Autodesk Inventor part; units mm, degrees
ref_plane "YZ Plane" through (0, 0, 0) normal (1, 0, 0) x (0, 1, 0)
ref_plane "XZ Plane" through (0, 0, 0) normal (0, 1, 0) x (-1, 0, 0)
ref_plane "XY Plane" through (0, 0, 0) normal (0, 0, 1) x (1, 0, 0)
sketch "スケッチ1" plane through (0, 0, 0) normal (0, 0, 1) x (1, 0, 0)
  line L0 (-5.9, -14.9) -> (5.9, -14.9) construction
  line L1 (5.9, -14.9) -> (5.9, 14.9) construction
  line L2 (5.9, 14.9) -> (-5.9, 14.9) construction
  line L3 (-5.9, 14.9) -> (-5.9, -14.9) construction
  line L4 (-5.9, -14.9) -> (5.9, 14.9) construction
  line L5 (5.9, -14.9) -> (-5.9, 14.9) construction
  circle A0 centre (-5.9, 14.9) radius 1.1
  circle A1 centre (-5.9, 14.9) radius 2
  circle A2 centre (5.9, 14.9) radius 2
  circle A3 centre (5.9, 14.9) radius 1.1
  circle A4 centre (-5.9, -14.9) radius 2
  circle A5 centre (-5.9, -14.9) radius 1.1
  circle A6 centre (5.9, -14.9) radius 2
  circle A7 centre (5.9, -14.9) radius 1.1
  circle A8 centre (0, 8.9998) radius 6.5
  circle A9 centre (-5.9, 14.9) radius 8.344 construction
  line L6 (-6.5, 8.9998) -> (6.5, 8.9998)
  line L7 (6.5, 8.9998) -> (6.5, -11.9)
  line L8 (6.5, -11.9) -> (-6.5, -11.9)
  line L9 (-6.5, -11.9) -> (-6.5, 8.9998)
  line L10 (-7.9, -16.9) -> (7.9, -16.9)
  line L11 (7.9, -16.9) -> (7.9, 16.9)
  line L12 (7.9, 16.9) -> (-7.9, 16.9)
  line L13 (-7.9, 16.9) -> (-7.9, -16.9)
  line L14 (-7.9, -16.9) -> (7.9, 16.9) construction
  line L15 (7.9, -16.9) -> (-7.9, 16.9) construction
  line L16 (-15.25, -0.0002) -> (15.25, -0.0002)
  line L17 (15.25, -0.0002) -> (15.25, 17.9998)
  line L18 (15.25, 17.9998) -> (-15.25, 17.9998)
  line L19 (-15.25, 17.9998) -> (-15.25, -0.0002)
  line L20 (-15.25, -0.0002) -> (15.25, 17.9998) construction
  line L21 (15.25, -0.0002) -> (-15.25, 17.9998) construction
  point P0 (0, 0)
  point P1 (0, 14.9)
  point P2 (7.9, -0.0002)
  point P3 (-7.9, -0.0002)
  point P4 (-7.9, -14.9)
  point P5 (-5.9, -16.9)
  point P6 (5.9, -16.9)
  point P7 (7.9, -14.9)
  point P8 (6.5, 8.9998)
  dimension "d12" = 13
  dimension "d13" = 16.688
  dimension "d0" = 11.8
  dimension "d1" = 29.8
  dimension "d2" = 2.2
  dimension "d3" = 4
  dimension "d6" = 11.8
  dimension "d9" = 29.8
  dimension "d14" = 3
  dimension "d15" = 30.5
  dimension "d16" = 18
extrude "押し出し1" add sketch "スケッチ1" along normal blind 3 contours A1 A8 | A1 L12 A2 A8 | L12 L13 L16 L19 L18 L17 L11 | A1 L13 L12 | A1 A8 L9 L16 L13 | L12 L11 A2 | A2 A8 | L16 L9 L8 L7 L11 A6 L10 A4 L13 | L11 L16 L7 A8 A2 | A4 | A6 picked at (-7.5833, 15.0483) picked at (7.5833, 15.0483)
fillet "フィレット1" radius 2 4 edges at (-7.9, -0.0002, 1.5) (7.9, -0.0002, 1.5) (-6.5, -11.9, 1.5) (6.5, -11.9, 1.5)
sketch "スケッチ2" plane through (-15.25, -0.0002, 0) normal (-1, 0, 0) x (0, 0, 1)
  line L0 (0, 18) -> (3, 18) construction
  line L1 (1.5, 18) -> (1.5, 0) construction
  line L2 (0, 0) -> (3, 0) construction
  line L3 (0, 9) -> (3, 9) construction
  line L4 (1.5, 9) -> (3, 9) construction
  point P0 (0, 0.0002)
  point P1 (1.5, 16.5)
  point P2 (1.5, 1.5)
  dimension "d20" = 15
hole "穴1" at (-15.25, 16.4998, 1.5) at (-15.25, 1.4998, 1.5) direction (1, 0, 0) diameter 1.567 depth 4.5 tip angle 118
sketch "スケッチ3" plane through (15.25, -0.0002, 0) normal (1, 0, 0) x (0, 0, -1)
  line L0 (0, 0) -> (0, 18)
  circle A0 centre (-1.5, 1.5) radius 0.7835
  circle A1 centre (-1.5, 16.5) radius 0.7835
  line L1 (0, 18) -> (0, 0)
  line L2 (0, 0) -> (-3, 0)
  line L3 (-3, 18) -> (-3, 0)
  line L4 (0, 18) -> (-3, 18)
  point P0 (0, 0.0002)
hole "穴2" at (15.25, 1.4998, 1.5) at (15.25, 16.4998, 1.5) direction (-1, 0, 0) diameter 1.567 depth 4.5 tip angle 118
sketch "スケッチ4" plane through (0, 0, 3) normal (0, 0, 1) x (1, 0, 0)
  line L0 (-15.25, 0.7163) -> (-15.25, 2.2833)
  line L1 (-15.25, 15.7163) -> (-15.25, 17.2833)
  circle A0 centre (-16.15, 1.4998) radius 1.1
  line L2 (-15.25, 17.9998) -> (-15.25, -0.0002) construction
  line L3 (-15.25, 8.9998) -> (15.25, 8.9998) construction
  line L4 (15.25, -0.0002) -> (15.25, 17.9998) construction
  line L5 (15.25, 17.9998) -> (-15.25, 17.9998) construction
  line L6 (0, 17.9998) -> (0, 8.9998) construction
  circle A1 centre (-16.15, 16.4998) radius 1.1
  line L7 (15.25, 0.7163) -> (15.25, 2.2833)
  line L8 (15.25, 15.7163) -> (15.25, 17.2833)
  circle A2 centre (16.15, 1.4998) radius 1.1
  line L9 (15.25, 17.9998) -> (15.25, -0.0002) construction
  circle A3 centre (16.15, 16.4998) radius 1.1
  point P0 (0, 0)
  point P1 (-15.25, 1.4998)
  point P2 (15.25, 1.4998)
  dimension "d35" = 2.2
  dimension "d36" = 0.9
extrude "押し出し2" cut sketch "スケッチ4" against normal blind 3
equation "\"d6\" = d0"
equation "\"d9\" = d1"
properties part number "udeyo"
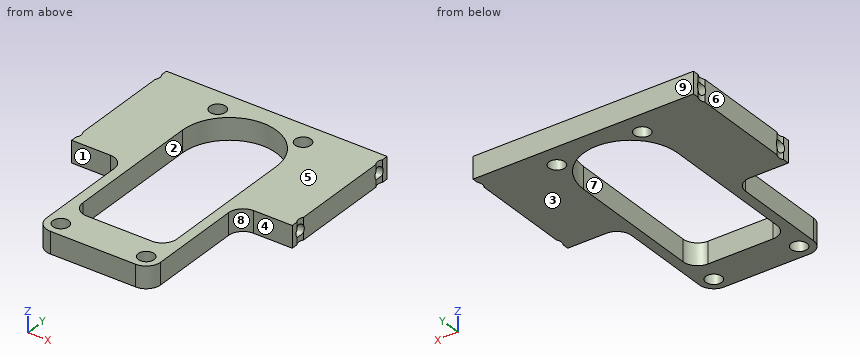
Design review of the part built by this model. Coordinates are the model's own, in mm. Face numbers are marked on the shaded views. A direction names the side the tool comes from. Coordinates: 2 decimals unless noted, no trailing zeros. Loops run counter-clockwise (first coordinate to the right, second up) from the corner with the lowest first, then second, coordinate; pieces in that order, holes last. Notation, with made-up numbers: (-25, 48.25) - (-12, 48.25) arc R9 cw to (-12, 60.25) - close; hole circle Ø2 at (-33, 12). An arc over 180 degrees is marked (long way). Use CSV: the item, a comma, the result in double quotes. Start each with the question number.
1) For pin 1 Ø2 at (x, y) = (-4, -7.5) entering from -Z; pin 2 Ø0.9 at (y, z) = (-7.5, 1.5) entering from +X, all flat-tipped, find the tip position at first contact; note any pin that passes through.
2) Consider section B-B on x = 0. Write out the cut boundary in (y, z).
3) The part is to be moulded in two halves that separate along Y. For the marked faces 6, 7, 8 and 9, say which applies: +Y half, -Y half, draft (parallel to the pull), parting line (faces both ways), or undercut.
4) Wall thickness on L1, parallel to Y at x = 12.3, z = 1.5; L2, parallel to X at y = -2, z = 1.05; L3, parallel to X at y = 0.5, z = 2.5: over which ranges is each line inside the solid? List them lowest first. Write a range as from..to.
5) Consider section A-A on y = 5. Write out the cut boundary in (x, z).
6) Tool access review of the marked faces 1, 2, 3, 4 and 5: name each direction out of +Z, -Z, +X, -X, +Y, -Y from which nothing blocks a thin tool from reaching the whole face with its end or side.
7) Consider section C-C on y = 14.9. Write out the cut boundary in (x, z), then the cut area to 3 significant figures.
Geometry says:
1,pin 1,"through"
1,pin 2,"x = 7.9"
2,outline,"(-16.9, 0) - (-11.9, 0) - (-11.9, 3) - (-16.9, 3) - close; (15.5, 0) - (18, 0) - (18, 3) - (15.5, 3) - close"
3,face 6,"draft"
3,face 7,"undercut"
3,face 8,"-Y half"
3,face 9,"+Y half"
4,L1,"0..0.72, 2.28..15.72, 17.28..18"
4,L2,"-7.9..-6.5, 6.5..7.9"
4,L3,"-15.25..-6.5, 6.5..15.25"
5,outline,"(-15.25, 0) - (-6.5, 0) - (-6.5, 3) - (-15.25, 3) - close; (6.5, 0) - (15.25, 0) - (15.25, 3) - (6.5, 3) - close"
6,face 1,"+Z, -Z, -X, -Y"
6,face 2,"+Z, -Z"
6,face 3,"-Z, +X, -X, +Y, -Y"
6,face 4,"+Z, -Z, +X, -Y"
6,face 5,"+Z, +X, -X, +Y, -Y"
7,outline,"(-15.25, 0) - (-7, 0) - (-7, 3) - (-15.25, 3) - close; (-4.8, 0) - (-2.73, 0) - (-2.73, 3) - (-4.8, 3) - close; (2.73, 0) - (4.8, 0) - (4.8, 3) - (2.73, 3) - close; (7, 0) - (15.25, 0) - (15.25, 3) - (7, 3) - close"
7,area,"61.9 mm^2"
